```python
from build123d import *

# Parameters (mm, degrees)
F0_R     = 3.2565865512
F1_DEPTH = 6.35


with BuildPart() as f1:
    # F0 (on Top) → F1 (new body)
    with BuildSketch(Plane.XY):
        with BuildLine():
            Line((-7.6721920632, 36.7054540553), (-7.6721920632, 37.0963104069))
            Line((-7.6721920632, 37.0963104069), (-2.9508429579, 37.0963104069))
            ThreePointArc((-2.9508429579, 37.0963104069), (-1.4615430474, 38.7866806162), (-0.9243947942, 40.9745648503))
            ThreePointArc((-0.9243947942, 40.9745648503), (-8.174638541, 44.9669975349), (-7.6721920632, 36.7054540553))
        make_face()
        with Locations((-5.6487568654, 40.9745648503)):
            Circle(F0_R, mode=Mode.SUBTRACT)
        with BuildLine():
            Line((-2.9508429579, 37.0963104069), (-7.6721920632, 37.0963104069))
            Line((-7.6721920632, 37.0963104069), (-7.6721920632, 36.7054540553))
            ThreePointArc((-7.6721920632, 36.7054540553), (-5.2589844262, 36.2663088648), (-2.9508429579, 37.0963104069))
        make_face()
        with BuildLine():
            Line((-2.9508429579, 0), (-2.9508429579, 37.0963104069))
            ThreePointArc((-2.9508429579, 37.0963104069), (-5.2589844262, 36.2663088648), (-7.6721920632, 36.7054540553))
            Line((-7.6721920632, 36.7054540553), (-7.6721920632, 0))
            Line((-7.6721920632, 0), (-2.9508429579, 0))
        make_face()
    extrude(amount=F1_DEPTH)


solid = f1.part
```
Input: part model. Units: mm. Frame: model coordinates. A direction names the side the tool comes from. Round coordinates to 2 decimals unless told otherwise and drop trailing zeros. Order: outer loops, then holes, each group sorted by start corner. A loop starts at its lowest first (then second) coordinate and runs counter-clockwise, first axis right, second up. Notation, with made-up numbers: (17, 52.25) - (40, 52.25) arc R23 cw to (40, 75.25) - close; hole circle Ø2 at (67.25, 18.25). An arc over 180 degrees is marked (long way). Answer in a Markdown table with one row per item.
Item 1: Mould query, pull axis Z, two halves, no side actions, for faces 1 (the flat face through (-5, 0, 3)), 2 (the flat face through (-6, 23, 6.35)), 3 (the flat face through (-6, 23, 0)). Classes: released by +Z, released by -Z, zero draft, split by the parting line, or undercut.
Model answer:
| item | result |
|---|---|
| face 1 | zero draft |
| face 2 | released by +Z |
| face 3 | released by -Z |
Item 2: Section query D-D (y = 4.5). Return the cut outline in (x, z).
Model answer:
| item | result |
|---|---|
| outline | (-7.67, 0) - (-2.95, 0) - (-2.95, 6.35) - (-7.67, 6.35) - close |
Item 3: Section query C-C (z = 1.75). Return the cut outline in (x, y).
Model answer:
| item | result |
|---|---|
| outline | (-7.67, 0) - (-2.95, 0) - (-2.95, 37.1) arc R4.72 ccw (long way) to (-7.67, 36.71) - close; hole circle Ø6.51 at (-5.65, 40.97) |
Item 4: Line query: line 1 (Y direction, x = -5.75, z = 3); line 2 (X direction, y = 41, z = 4); line 3 (X direction, y = 13.5, z = 4.75). Output: solid intervals per line, ascending.
Model answer:
| item | result |
|---|---|
| line 1 | y = 0 to 37.72, 44.23 to 45.7 |
| line 2 | x = -10.37 to -8.91, -2.39 to -0.92 |
| line 3 | x = -7.67 to -2.95 |
Item 5: Pin query (flat end, axial travel): pin 1 (4 mm diameter, centred on x = -5.65, y = 40.97, fed in from +Z); pin 2 (1.9 mm diameter, centred on y = 12, z = 3, fed in from -X); pin 3 (1 mm diameter, centred on y = 10, z = 5.5, fed in from +X). Return the tip coordinate at first contact, or that it passes through.
Model answer:
| item | result |
|---|---|
| pin 1 | passes through |
| pin 2 | stops at x = -7.67 |
| pin 3 | stops at x = -2.95 |
Item 6: Section query A-A (x = -7). Return the cut outline in (y, z).
Model answer:
| item | result |
|---|---|
| outline | (0, 0) - (38.01, 0) - (38.01, 6.35) - (0, 6.35) - close; (43.94, 0) - (45.5, 0) - (45.5, 6.35) - (43.94, 6.35) - close |
Item 7: Section query B-B (y = 42). Return the cut outline in (x, z).
Model answer:
| item | result |
|---|---|
| outline | (-10.26, 0) - (-8.74, 0) - (-8.74, 6.35) - (-10.26, 6.35) - close; (-2.56, 0) - (-1.04, 0) - (-1.04, 6.35) - (-2.56, 6.35) - close |
Item 8: Reachability of faces 4 (the flat face through (-7.672, 19, 3)), 5 (the cylindrical face through (-6.355, 37.795, 3.131)), 6 (the flat face through (-2.951, 18, 3)) from +Z, -Z, +X, -X, +Y, -Y: full face, straight path, thin tool, end or side. Return the list, or none.
Model answer:
| item | result |
|---|---|
| face 4 | +Z, -Z, -X, -Y |
| face 5 | +Z, -Z |
| face 6 | +Z, -Z, +X, -Y |
